```python
from build123d import *

# Parameters (mm, degrees)
BOSS_EXTRUDE1_DEPTH     = 7.5
F_1_4_CLEARANCE_HOLE4_D = 6.5278
M4_CLEARANCE_HOLE1_D    = 4.3


with BuildPart() as part:
    # Sketch2 → Boss-Extrude1 (new body)
    with BuildSketch(Plane(origin=(0, 0, 0), x_dir=(1, 0, 0), z_dir=(0, 1, 0))):
        with BuildLine():
            Line((0, 0), (140, 0))
            ThreePointArc((140, 0), (147.071067812, 2.928932188), (150, 10))
            Line((150, 10), (150, 43.095020321))
            ThreePointArc((150, 43.095020321), (148.228885216, 48.777048841), (143.54291038, 52.446372418))
            Line((143.54291038, 52.446372418), (3.54291038, 105.487627635))
            ThreePointArc((3.54291038, 105.487627635), (0, 106.136275538), (-3.54291038, 105.487627635))
            Line((-3.54291038, 105.487627635), (-143.54291038, 52.446372418))
            ThreePointArc((-143.54291038, 52.446372418), (-148.228885216, 48.777048841), (-150, 43.095020321))
            Line((-150, 43.095020321), (-150, 10))
            ThreePointArc((-150, 10), (-147.071067812, 2.928932188), (-140, 0))
            Line((-140, 0), (0, 0))
        make_face()
    extrude(amount=-BOSS_EXTRUDE1_DEPTH)

    # 1/4 Clearance Hole4 (through all)
    with Locations(Plane(origin=(0, 0, 0), x_dir=(1, 0, 0), z_dir=(0, 1, 0))):
        with Locations((84.499767088, 28.031140011), (-84.499767088, 28.031140011), (0, 40), (0, 20)):
            Hole(F_1_4_CLEARANCE_HOLE4_D / 2)

    # M4 Clearance Hole1 (through all)
    with Locations(Plane(origin=(0, 0, 0), x_dir=(1, 0, 0), z_dir=(0, 1, 0))):
        with Locations((-76.49119694, 41.758956585), (-99.869577175, 32.901680638), (76.49119694, 41.758956585), (99.869577175, 32.901680638)):
            Hole(M4_CLEARANCE_HOLE1_D / 2)


solid = part.part
```
Can you work these out from the model? Positions are in its coordinate system, mm. Coordinates: 2 decimals unless noted, no trailing zeros. Loops run counter-clockwise (first coordinate to the right, second up) from the corner with the lowest first, then second, coordinate; pieces in that order, holes last.
Item 1: Suppose I cut it at D-D (z = -67.5). Please give me the cut outline in (x, y), then the cut area to 3 significant figures.
Answers below:
outline: (-103.81, -7.5) - (103.81, -7.5) - (103.81, 0) - (-103.81, 0) - close
area: 1,560 mm2
Item 2: Suppose I cut it at A-A (z = -20). Please give me the cut outline in (x, y).
Answers below:
outline: (-150, -7.5) - (-3.26, -7.5) - (-3.26, 0) - (-150, 0) - close; (3.26, -7.5) - (150, -7.5) - (150, 0) - (3.26, 0) - close
Item 3: Please list where these lines run through material, in increasing order: L1, parallel to X at y = -3.75, z = -32.5; L2, parallel to Z at x = 0, y = -1.25; L3, parallel to X at y = -2.75, z = -28.
Answers below:
L1: x = -150 to -101.98, -97.76 to 97.76, 101.98 to 150
L2: z = -106.14 to -43.26, -36.74 to -23.26, -16.74 to 0
L3: x = -150 to -87.76, -81.24 to 81.24, 87.76 to 150
Item 4: Suppose I cut it at B-B (x = 0). Please give me the cut outline in (y, z).
Answers below:
outline: (-7.5, -106.14) - (0, -106.14) - (0, -43.26) - (-7.5, -43.26) - close; (-7.5, -36.74) - (0, -36.74) - (0, -23.26) - (-7.5, -23.26) - close; (-7.5, -16.74) - (0, -16.74) - (0, 0) - (-7.5, 0) - close
Item 5: I'm going to push flat-ended pins straight in: pin 1 (2 mm diameter, centred on x = -31, y = -3.5, fed in from -Z); pin 2 (1.5 mm diameter, centred on x = -37.5, y = -3.5, fed in from -Z). Where does each tip first touch, or does it pass through?
Answers below:
pin 1: stops at z = -95.46
pin 2: stops at z = -92.91
Item 6: If we mould it in two halves opening along Z, with no side actions, what happens to faces 1 (the face through (0.051, -3.698, -106.136)), 2 (the face through (-150, -4, -27)), 3 (the face through (0.708, -3.803, -36.814))? For each: released by +Z, released by -Z, zero draft, split by the parting line, or undercut.
Answers below:
face 1: released by -Z
face 2: zero draft
face 3: undercut
Item 7: Suppose I cut it at C-C (y = -6.25). State how many separate pieces and enclosed holes the cut face has, then the cut area to 3 significant figures.
Answers below:
separate pieces: 1
enclosed holes: 8
area: 23,300 mm2
